from build123d import *

# Parameters (mm, degrees)
BOSS_EXTRU_1_DEPTH      = 3
ESQUISSE2_R             = 1.5
ENL_V_MAT_EXTRU_1_DEPTH = 95.249668434
ESQUISSE3_R             = 2
ESQUISSE3_R_2           = 1.5
ENL_V_MAT_EXTRU_2_DEPTH = 95.249668434
CONG_1_R                = 3
ESQUISSE4_R             = 1.5
ENL_V_MAT_EXTRU_3_DEPTH = 95.249668434


with BuildPart() as part:
    # Esquisse1 → Boss.-Extru.1 (new body)
    with BuildSketch(Plane.XY):
        Polygon((0, 0), (75, 0), (75, 57), (40, 57), (25, 27), (0, 27), align=None)
    extrude(amount=BOSS_EXTRU_1_DEPTH)

    # Esquisse2 → Enlèv. mat.-Extru.1 (cut, through all)
    with BuildSketch(Plane.XY.offset(3)):
        with Locations((42, 37)):
            Circle(ESQUISSE2_R)
        with Locations(Location((42, 13, 0), (0, 0, 180))):
            Circle(ESQUISSE2_R)
        with Locations((65, 13)):
            Circle(ESQUISSE2_R)
        with Locations(Location((65, 37, 0), (0, 0, 180))):
            Circle(ESQUISSE2_R)
    extrude(amount=-ENL_V_MAT_EXTRU_1_DEPTH, mode=Mode.SUBTRACT)

    # Esquisse3 → Enlèv. mat.-Extru.2 (cut, through all)
    with BuildSketch(Plane.XY.offset(3)):
        with Locations((5, 22)):
            Circle(ESQUISSE3_R)
        with Locations((5, 5)):
            Circle(ESQUISSE3_R)
        with Locations((52.5, 3)):
            Circle(ESQUISSE3_R_2)
        with Locations((52.5, 54)):
            Circle(ESQUISSE3_R_2)
        with Locations((72, 37)):
            Circle(ESQUISSE3_R_2)
    extrude(amount=-ENL_V_MAT_EXTRU_2_DEPTH, mode=Mode.SUBTRACT)

    # Congé1
    cong_1_edges = [part.edges().sort_by_distance(p)[0] for p in [
        (0, 27, 1.5),
        (25, 27, 1.5),
        (40, 57, 1.5),
        (75, 57, 1.5),
        (75, 0, 1.5),
        (0, 0, 1.5),
    ]]
    fillet(cong_1_edges, radius=CONG_1_R)

    # Esquisse4 → Enlèv. mat.-Extru.3 (cut, through all)
    with BuildSketch(Plane.XY.offset(3)):
        with Locations((26, 21)):
            Circle(ESQUISSE4_R)
        with Locations((26, 9)):
            Circle(ESQUISSE4_R)
    extrude(amount=-ENL_V_MAT_EXTRU_3_DEPTH, mode=Mode.SUBTRACT)


solid = part.part
Geometry: final body of the model. Coordinates: model frame, mm. A direction names the side the tool comes from. Give positions to 0.01 mm unless a question says otherwise; leave off trailing zeros. Order: outer loops, then holes, each group sorted by start corner. A loop starts at its lowest first (then second) coordinate and runs counter-clockwise, first axis right, second up. Notation, with made-up numbers: (2, -7.5) -> (24, -7.5) arc R6 ccw to (24, 3.5) -> close; hole circle Ø10 at (9.25, 71). An arc over 180 degrees is marked (long way). Put each result on its own line as item: value.
Q1. Material intervals for L1, parallel to Y at x = 42, z = 1.8; L2, parallel to Y at x = 26, z = 0.75; L3, parallel to Y at x = 17, z = 1.3, sorted ascending.
Here are the results:
L1: y = 0 to 11.5, 14.5 to 35.5, 38.5 to 57
L2: y = 0 to 7.5, 10.5 to 19.5, 22.5 to 29
L3: y = 0 to 27
Q2. Section B-B, the plane y = 13. Return loops of the section in (x, z).
Here are the results:
outline: (0, 0) -> (40.5, 0) -> (40.5, 3) -> (0, 3) -> close; (43.5, 0) -> (63.5, 0) -> (63.5, 3) -> (43.5, 3) -> close; (66.5, 0) -> (75, 0) -> (75, 3) -> (66.5, 3) -> close
Q3. Section D-D, the plane y = 50. Return loops of the section in (x, z).
Here are the results:
outline: (36.5, 0) -> (75, 0) -> (75, 3) -> (36.5, 3) -> close
Q4. Pin query (flat end, axial travel): pin 1 (0.9 mm diameter, centred on x = 12, z = 1.5, fed in from +Y); pin 2 (3 mm diameter, centred on x = 5, y = 5, fed in from -Z). Return the tip coordinate at first contact, or that it passes through.
Here are the results:
pin 1: stops at y = 27
pin 2: passes through
Q5. Section A-A, the plane x = 52.5. Return loops of the section in (y, z).
Here are the results:
outline: (0, 0) -> (1.5, 0) -> (1.5, 3) -> (0, 3) -> close; (4.5, 0) -> (52.5, 0) -> (52.5, 3) -> (4.5, 3) -> close; (55.5, 0) -> (57, 0) -> (57, 3) -> (55.5, 3) -> close
Q6. Reachability of faces 1 (the face through (13, 27, 1)), 2 (the face through (3.4, 20.8, 1.5)) from +Z, -Z, +X, -X, +Y, -Y: full face, straight path, thin tool, end or side. Return the list, or none.
Here are the results:
face 1: +Z, -Z, -X, +Y
face 2: +Z, -Z
Q7. Draft query along X for faces 3 (the face through (24.89, 22.01, 1.52)), 4 (the face through (43.5, 12.93, 1.52)), 5 (the face through (74.14, 56.1, 1.52)), 6 (the face through (32.6, 42.2, 1.5)). Return one class per face: released by +X, released by -X, zero draft, split by the parting line, or undercut.
Here are the results:
face 3: undercut
face 4: undercut
face 5: released by +X
face 6: released by -X
Q8. Section C-C, the plane z = 0.7. Count the separate pieces of the cut face and the enclosed holes in it, then the cut area to 3 significant figures.
Here are the results:
separate pieces: 1
enclosed holes: 11
area: 3,200 mm^2
